Read the model definition and answer for the solid it produces. Units are mm, in the model's axes. A direction names the side the tool comes from. Coordinates: 2 decimals unless noted, no trailing zeros. Order: outer loops, then holes, each group sorted by start corner. A loop starts at its lowest first (then second) coordinate and runs counter-clockwise, first axis right, second up. Notation, with made-up numbers: (-9, 84.5) - (46, 84.5) arc R27 cw to (46, 101.5) - close; hole circle Ø11 at (-37, -7). An arc over 180 degrees is marked (long way). Use one line per item in the form item = value. Start each with the question number.
from build123d import *

# Parameters (mm, degrees)
BOSS_EXTRUDE1_DEPTH          = 28.5
SKETCH2_R                    = 21
BOSS_EXTRUDE2_DEPTH          = 32
SKETCH3_R                    = 22
BOSS_EXTRUDE3_DEPTH          = 32
SKETCH4_R                    = 21.35
BOSS_EXTRUDE4_DEPTH          = 8
SKETCH5_R                    = 20.85
BOSS_EXTRUDE5_DEPTH          = 36
SKETCH6_W                    = 28
SKETCH6_H                    = 28.5
BOSS_EXTRUDE6_DEPTH          = 21.22463282
SKETCH7_R                    = 21.1
BOSS_EXTRUDE7_DEPTH          = 8
SKETCH8_R                    = 13.3
BOSS_EXTRUDE8_DEPTH          = 2
SKETCH9_R                    = 4
BOSS_EXTRUDE9_DEPTH          = 20
CUT_EXTRUDE1_DEPTH           = 12
CUT_EXTRUDE2_DEPTH           = 15
F_4_0_4_DIAMETER_HOLE1_D     = 4
F_4_0_4_DIAMETER_HOLE1_DEPTH = 2


with BuildPart() as part:
    # Sketch1 → Boss-Extrude1 (new body)
    with BuildSketch(Plane(origin=(0, 0, 0), x_dir=(-1, 0, 0), z_dir=(0, 0, -1))):
        with BuildLine():
            Line((14.707413083, 18.007068068), (14.707413083, 19.07536718))
            Line((14.707413083, 19.07536718), (-13.292586917, 19.07536718))
            ThreePointArc((-13.292586917, 19.07536718), (-0.886424853, -23.233096027), (14.707413083, 18.007068068))
        make_face()
    extrude(amount=-BOSS_EXTRUDE1_DEPTH)

    # Sketch2 → Boss-Extrude2 (add)
    with BuildSketch(Plane.XY.offset(28.5)):
        Circle(SKETCH2_R)
    extrude(amount=BOSS_EXTRUDE2_DEPTH)

    # Sketch3 → Boss-Extrude3 (add)
    with BuildSketch(Plane(origin=(0, 0, 60.5), x_dir=(-1, 0, 0), z_dir=(0, 0, -1))):
        Circle(SKETCH3_R)
    extrude(amount=-BOSS_EXTRUDE3_DEPTH)

    # Sketch4 → Boss-Extrude4 (add)
    with BuildSketch(Plane.XY.offset(92.5)):
        Circle(SKETCH4_R)
    extrude(amount=BOSS_EXTRUDE4_DEPTH)

    # Sketch5 → Boss-Extrude5 (add)
    with BuildSketch(Plane.XY.offset(100.5)):
        Circle(SKETCH5_R)
    extrude(amount=BOSS_EXTRUDE5_DEPTH)

    # Sketch6 → Boss-Extrude6 (add)
    with BuildSketch(Plane(origin=(0, 19.07536718, 0), x_dir=(-1, 0, 0), z_dir=(0, 1, 0))):
        with Locations((0.707413083, 14.25)):
            Rectangle(SKETCH6_W, SKETCH6_H)
    extrude(amount=BOSS_EXTRUDE6_DEPTH)

    # Sketch7 → Boss-Extrude7 (add)
    with BuildSketch(Plane(origin=(0, 0, 136.5), x_dir=(-1, 0, 0), z_dir=(0, 0, -1))):
        Circle(SKETCH7_R)
    extrude(amount=-BOSS_EXTRUDE7_DEPTH)

    # Sketch8 → Boss-Extrude8 (add)
    with BuildSketch(Plane.XY.offset(144.5)):
        Circle(SKETCH8_R)
    extrude(amount=BOSS_EXTRUDE8_DEPTH)

    # Sketch9 → Boss-Extrude9 (add)
    with BuildSketch(Plane.XY.offset(146.5)):
        Circle(SKETCH9_R)
    extrude(amount=BOSS_EXTRUDE9_DEPTH)

    # Sketch10 → Cut-Extrude1 (cut)
    with BuildSketch(Plane.XY.offset(166.5)):
        with BuildLine():
            Line((-3.255366619, 2.324346828), (3.255366619, 2.324346828))
            ThreePointArc((3.255366619, 2.324346828), (0, 4), (-3.255366619, 2.324346828))
        make_face()
    extrude(amount=-CUT_EXTRUDE1_DEPTH, mode=Mode.SUBTRACT)

    # Sketch11 → Cut-Extrude2 (cut)
    with BuildSketch(Plane.XY.offset(28.5)):
        with BuildLine():
            Line((10.960399944, 19.07536718), (10.960399944, 37.965647442))
            Line((10.960399944, 37.965647442), (-12.639046626, 37.965647442))
            Line((-12.639046626, 37.965647442), (-12.639046626, 18.007068068))
            ThreePointArc((-12.639046626, 18.007068068), (-0.994876585, 21.977493501), (10.960399944, 19.07536718))
        make_face()
    extrude(amount=-CUT_EXTRUDE2_DEPTH, mode=Mode.SUBTRACT)

    # Ø4.0 (4) Diameter Hole1
    with Locations(Plane.XY.offset(144.5)):
        with Locations((-13.043990964, -12.610936722), (12.610936722, -13.043990964), (13.043990964, 12.610936722), (-12.610936722, 13.043990964)):
            Hole(F_4_0_4_DIAMETER_HOLE1_D / 2, depth=F_4_0_4_DIAMETER_HOLE1_DEPTH)


solid = part.part
Q1. A cutting plane is placed at D-D (y = 26.5). Give the vertices of the cut face in (x, z).
Q2. Consider probe 1 along Z at (x, y) = (-11, 19); probe 2 along Z at (x, y) = (1.5, 31); probe 3 along Z at (x, y) = (8, -2.5). Determine where each line is inside the solid, lowest interval first.
Q3. For a pull along X with two mould halves and no side action, classify faces 4 (the cylindrical face through (20.03, 6.31, 44.28)), 5 (the flat face through (20.5, -4.6, 100.5)), 6 (the cylindrical face through (11.97, 14.3, 143.49)) as +X half, -X half, draft (parallel to the pull), parting line (faces both ways), or undercut.
Q4. Given P1, Ø1.2, axis at x = -13, y = -11.5, coming from the +Z side; P2, Ø24.5, axis at y = 29.5, z = 12, coming from the -X side; P3, Ø3, axis at x = -10, y = -14.5, coming from the +Z side, each flat-ended and moving along its own axis, determine where each tip first touches the part or whether it passes through.
Q5. Which of the six approach directions +Z, -Z, +X, -X, +Y, -Y give full straight-line access (tool end or side, diameter ignored) to faces 1 (the cylindrical face through (-13.967, -14.385, 143.486)), 2 (the flat face through (0, -1, 166.5)), 3 (the flat face through (-7, 20, 28.5))?
Q6. A cutting plane is placed at B-B (z = 96). Give the vertices of the cut face in (x, y).
Result sheet:
q1.outline = (-14.71, 0) - (13.29, 0) - (13.29, 28.5) - (10.96, 28.5) - (10.96, 13.5) - (-12.64, 13.5) - (-12.64, 28.5) - (-14.71, 28.5) - close
q2.probe_1 = 0 to 28.5, 60.5 to 92.5
q2.probe_2 = 0 to 13.5
q2.probe_3 = 0 to 146.5
q3.face_4 = parting line
q3.face_5 = draft
q3.face_6 = undercut
q4.P1 = 142.5
q4.P2 = -15.59
q4.P3 = 144.5
q5.face_1 = +Z
q5.face_2 = +Z, +X, -X, +Y, -Y
q5.face_3 = none
q6.outline = circle Ø42.7 at (0, 0)
